```python
from build123d import *

# Parameters (mm, degrees)
BOSS_EXTRUDE2_DEPTH = 96
SKETCH4_W           = 10
SKETCH4_H           = 96
SKETCH4_R           = 2.25
BOSS_EXTRUDE3_DEPTH = 3.5
BOSS_EXTRUDE4_START = -5
BOSS_EXTRUDE4_DEPTH = 5
SKETCH6_R           = 2.125
CUT_EXTRUDE1_DEPTH  = 5
SKETCH7_R           = 7.5
CUT_EXTRUDE2_DEPTH  = 97
SKETCH8_W           = 55
SKETCH8_H           = 25.5
CUT_EXTRUDE3_DEPTH  = 47.5
FILLET1_R           = 1


with BuildPart() as part:
    # Sketch1 → Boss-Extrude2 (new body)
    with BuildSketch(Plane.XY):
        with BuildLine():
            Line((-27.5, -22.5), (-27.5, 0))
            ThreePointArc((-27.5, 0), (0, 27.5), (27.5, 0))
            Line((27.5, 0), (27.5, -22.5))
            Line((27.5, -22.5), (17.5, -22.5))
            Line((17.5, -22.5), (17.5, -14.142135624))
            ThreePointArc((17.5, -14.142135624), (0, 22.5), (-17.5, -14.142135624))
            Line((-17.5, -14.142135624), (-17.5, -22.5))
            Line((-17.5, -22.5), (-27.5, -22.5))
        make_face()
    extrude(amount=BOSS_EXTRUDE2_DEPTH)

    # Sketch4 → Boss-Extrude3 (add)
    with BuildSketch(Plane.XZ.offset(22.5)):
        with Locations((-32.5, 48)):
            Rectangle(SKETCH4_W, SKETCH4_H)
        with Locations((-32.5, 91)):
            Circle(SKETCH4_R, mode=Mode.SUBTRACT)
        with Locations((-32.5, 5)):
            Circle(SKETCH4_R, mode=Mode.SUBTRACT)
        with Locations((32.5, 48)):
            Rectangle(SKETCH4_W, SKETCH4_H)
        with Locations((32.5, 5)):
            Circle(SKETCH4_R, mode=Mode.SUBTRACT)
        with Locations((32.5, 91)):
            Circle(SKETCH4_R, mode=Mode.SUBTRACT)
    extrude(amount=-BOSS_EXTRUDE3_DEPTH)

    # Sketch5 → Boss-Extrude4 (add)
    with BuildSketch(Plane.XY.offset(96).offset(BOSS_EXTRUDE4_START)):
        with BuildLine():
            Line((-27.5, -19), (-27.5, 0))
            ThreePointArc((-27.5, 0), (0, 27.5), (27.5, 0))
            Line((27.5, 0), (27.5, -19))
            Line((27.5, -19), (27.5, -22.5))
            Line((27.5, -22.5), (-27.5, -22.5))
            Line((-27.5, -22.5), (-27.5, -19))
        make_face()
    extrude(amount=BOSS_EXTRUDE4_DEPTH)

    # Sketch6 → Cut-Extrude1 (cut)
    with BuildSketch(Plane.XY.offset(96)):
        with Locations((-7.541666667, 13.06254984)):
            Circle(SKETCH6_R)
        with Locations((7.541666667, 13.06254984)):
            Circle(SKETCH6_R)
        with Locations((15.083333333, 0)):
            Circle(SKETCH6_R)
        with Locations((7.541666667, -13.06254984)):
            Circle(SKETCH6_R)
        with Locations((-7.541666667, -13.06254984)):
            Circle(SKETCH6_R)
        with Locations((-15.083333333, 0)):
            Circle(SKETCH6_R)
    extrude(amount=-CUT_EXTRUDE1_DEPTH, mode=Mode.SUBTRACT)

    # Sketch7 → Cut-Extrude2 (cut, through all)
    with BuildSketch(Plane.XY.offset(96)):
        Circle(SKETCH7_R)
    extrude(amount=-CUT_EXTRUDE2_DEPTH, mode=Mode.SUBTRACT)

    # Sketch8 → Cut-Extrude3 (cut, through all)
    with BuildSketch(Plane(origin=(0, -19, 0), x_dir=(1, 0, 0), z_dir=(0, 1, 0))):
        with Locations((0, -27.75)):
            Rectangle(SKETCH8_W, SKETCH8_H)
        with Locations((0, -68.25)):
            Rectangle(SKETCH8_W, SKETCH8_H)
    extrude(amount=CUT_EXTRUDE3_DEPTH, mode=Mode.SUBTRACT)

    # Fillet1
    fillet1_edges = [part.edges().sort_by_distance(p)[0] for p in [
        (-37.5, -20.75, 0),
        (-37.5, -20.75, 96),
        (37.5, -20.75, 96),
        (37.5, -20.75, 0),
    ]]
    fillet(fillet1_edges, radius=FILLET1_R)


solid = part.part
```
Can you work these out from the model? Positions are in its coordinate system, mm. A direction names the side the tool comes from. Round coordinates to 2 decimals unless told otherwise and drop trailing zeros. Loops run counter-clockwise (first coordinate to the right, second up) from the corner with the lowest first, then second, coordinate; pieces in that order, holes last.
Item 1: Please list where these lines run through material, in increasing order: L1, parallel to Z at x = 18, y = 16; L2, parallel to Z at x = -32.5, y = -20.4; L3, parallel to Y at x = 24.5, z = 39.
Item 2: Suppose I cut it at D-D, the plane z = 79. Write out the boundary of the cut face in (x, y), then the cut area to 3 significant figures.
Item 3: If we mould it in two halves opening along X, with no side actions, what happens to faces 1 (the cylindrical face through (17.11, 0.64, 93.54)), 2 (the flat face through (-8.3, 21.4, 40.5)), 3 (the cylindrical face through (-0.605, 27.493, 47.895))? For each: +X half, -X half, draft (parallel to the pull), parting line (faces both ways), or undercut.
Item 4: Suppose I cut it at C-C, the plane y = 5. Write out the boundary of the cut face in (x, z).
Item 5: Suppose I cut it at B-B, the plane x = 0. Write out the boundary of the cut face in (y, z).
Item 6: Will these pins go through, and if not, where does the flat tip stop? pin 1 Ø5.5 at (x, y) = (7.54, 13.06) entering from -Z; pin 2 Ø7.5 at (y, z) = (-8, 5) entering from +X; pin 3 Ø2.5 at (x, z) = (-32.5, 5) entering from -Y; pin 4 Ø16.5 at (y, z) = (-7.5, 87) entering from -X.
Item 7: Which directions (+Z, -Z, +X, -X, +Y, -Y) give clear straight access to the entire face, cutting with the end or side of a thin tool? Please do faces 4 (the flat face through (-27.5, -10, 48)), 5 (the flat face through (27.5, -9, 48)), 6 (the cylindrical face through (0.71, 22.49, 7.4)).
Item 8: Suppose I cut it at A-A, the plane z = 5. Write out the boundary of the cut face in (x, y), then the cut area to 3 significant figures.
Reported:
1. L1: z = 0 to 15, 40.5 to 55.5, 81 to 96
1. L2: z = 0 to 2.75, 7.25 to 88.75, 93.25 to 96
1. L3: y = -22.5 to -19
2. outline: (-37.5, -22.5) - (-17.5, -22.5) - (-17.5, -19) - (-37.5, -19) - close; (17.5, -22.5) - (37.5, -22.5) - (37.5, -19) - (17.5, -19) - close
2. area: 140 mm2
3. face 1: undercut
3. face 2: draft
3. face 3: parting line
4. outline: (-27.04, 0) - (-21.94, 0) - (-21.94, 15) - (-27.04, 15) - close; (-27.04, 40.5) - (-21.94, 40.5) - (-21.94, 55.5) - (-27.04, 55.5) - close; (-27.04, 81) - (-21.94, 81) - (-21.94, 91) - (-5.59, 91) - (-5.59, 96) - (-27.04, 96) - close; (5.59, 91) - (21.94, 91) - (21.94, 81) - (27.04, 81) - (27.04, 96) - (5.59, 96) - close; (21.94, 0) - (27.04, 0) - (27.04, 15) - (21.94, 15) - close; (21.94, 40.5) - (27.04, 40.5) - (27.04, 55.5) - (21.94, 55.5) - close
5. outline: (-22.5, 91) - (-7.5, 91) - (-7.5, 96) - (-22.5, 96) - close; (7.5, 91) - (22.5, 91) - (22.5, 81) - (27.5, 81) - (27.5, 96) - (7.5, 96) - close; (22.5, 0) - (27.5, 0) - (27.5, 15) - (22.5, 15) - close; (22.5, 40.5) - (27.5, 40.5) - (27.5, 55.5) - (22.5, 55.5) - close
6. pin 1: stops at z = 91
6. pin 2: stops at x = 27.5
6. pin 3: passes through
6. pin 4: stops at x = -27.5
7. face 4: +Z, -Z, -X, +Y
7. face 5: +Z, -Z, +X, +Y
7. face 6: -Z
8. outline: (-37.5, -22.5) - (-34.75, -22.5) - (-34.75, -19) - (-37.5, -19) - close; (-30.25, -22.5) - (-17.5, -22.5) - (-17.5, -14.14) arc R22.5 cw (long way) to (17.5, -14.14) - (17.5, -22.5) - (30.25, -22.5) - (30.25, -19) - (27.5, -19) - (27.5, 0) arc R27.5 ccw to (-27.5, 0) - (-27.5, -19) - (-30.25, -19) - close; (34.75, -22.5) - (37.5, -22.5) - (37.5, -19) - (34.75, -19) - close
8. area: 785 mm2
